Here's how the part is built. I have some questions about the finished solid (model axes, mm). Face numbers are marked on the shaded views. A direction names the side the tool comes from. Coordinates: 2 decimals unless noted, no trailing zeros. Write each loop counter-clockwise with the first axis right and the second up, starting at its lowest first coordinate (ties: lowest second). Pieces come first, ordered by that corner, then holes.
(1) Which directions (+Z, -Z, +X, -X, +Y, -Y) give clear straight access to the entire face, cutting with the end or side of a thin tool? Please do the marked faces 1, 2 and 3.
(2) Imagine slicing it at C-C, the plane y = -7.5. List the corners of the cut face in (x, z) for me (3 decimals).
(3) Imagine slicing it at D-D, the plane x = 2. List the corners of the cut face in (y, z) for me.
(4) Imagine slicing it at A-A, the plane y = 16.5. List the corners of the cut face in (x, z) for me.
(5) Thinking about a two-plate mould opening in Z: for the marked faces 4, 5, 6 and 7, which applies, released by +Z, released by -Z, zero draft, split by the parting line, or undercut?
(6) Please list where these lines run through material, in increasing order: probe 1 along Y at (x, z) = (0.25, 3.5); probe 2 along Y at (x, z) = (0, 3.65); probe 3 along Z at (x, y) = (0.6, 16.5).
(7) Imagine slicing it at B-B, the plane z = 4.75. List the corners of the cut face in (x, y) for me.
(8) For pin 1 Ø3 at (y, z) = (15.5, 4.5) entering from -X; pin 2 Ø0.8 at (x, z) = (-2, 2) entering from +Y, each with a flat end and sliding along its axis, tell me the tip position at first contact or that it passes through.
```python
from build123d import *

# Parameters (mm, degrees)
BOSS_EXTRUDE1_DEPTH = 6
SKETCH2_R           = 1.6
CUT_EXTRUDE1_DEPTH  = 22.644860822
CUT_EXTRUDE2_DEPTH  = 2.5
SKETCH4_R           = 1.1
CUT_EXTRUDE3_DEPTH  = 22.828879953
CUT_EXTRUDE4_DEPTH  = 22.828879953
FILLET1_R           = 2


with BuildPart() as part:
    # Sketch1 → Boss-Extrude1 (new body)
    with BuildSketch(Plane.XY):
        Polygon((-1, 12.5), (-1, 20.5), (1, 20.5), (1, 12.5), (3.5, 12.5), (3.5, -12.5), (-3.5, -12.5), (-3.5, 12.5), align=None)
    extrude(amount=BOSS_EXTRUDE1_DEPTH)

    # Sketch2 → Cut-Extrude1 (cut, through all)
    with BuildSketch(Plane.XY.offset(6)):
        with Locations((0, -7.5)):
            Circle(SKETCH2_R)
    extrude(amount=-CUT_EXTRUDE1_DEPTH, mode=Mode.SUBTRACT)

    # Sketch3 → Cut-Extrude2 (cut)
    with BuildSketch(Plane(origin=(0, 0, 0), x_dir=(-1, 0, 0), z_dir=(0, 0, -1))):
        Polygon((0, -4.295706006), (-2.775, -5.897853003), (-2.775, -9.102146997), (0, -10.704293994), (2.775, -9.102146997), (2.775, -5.897853003), align=None)
    extrude(amount=-CUT_EXTRUDE2_DEPTH, mode=Mode.SUBTRACT)

    # Sketch4 → Cut-Extrude3 (cut, through all)
    with BuildSketch(Plane.ZY.offset(1)):
        with Locations(Location((3, 16.5, 0), (0, 0, 270))):
            Circle(SKETCH4_R)
    extrude(amount=-CUT_EXTRUDE3_DEPTH, mode=Mode.SUBTRACT)

    # Sketch5 → Cut-Extrude4 (cut, through all)
    with BuildSketch(Plane.ZY.offset(1)):
        with BuildLine():
            Line((6, 20.5), (3, 20.5))
            ThreePointArc((3, 20.5), (4.645751311, 20.145751311), (6, 19.145751311))
            Line((6, 19.145751311), (6, 20.5))
        make_face()
        with BuildLine():
            Line((0, 20.5), (0, 19.145751311))
            ThreePointArc((0, 19.145751311), (1.354248689, 20.145751311), (3, 20.5))
            Line((3, 20.5), (0, 20.5))
        make_face()
    extrude(amount=-CUT_EXTRUDE4_DEPTH, mode=Mode.SUBTRACT)

    # Fillet1
    fillet1_edges = [part.edges().sort_by_distance(p)[0] for p in [
        (3.5, -12.5, 3),
        (-3.5, -12.5, 3),
    ]]
    fillet(fillet1_edges, radius=FILLET1_R)


solid = part.part
```
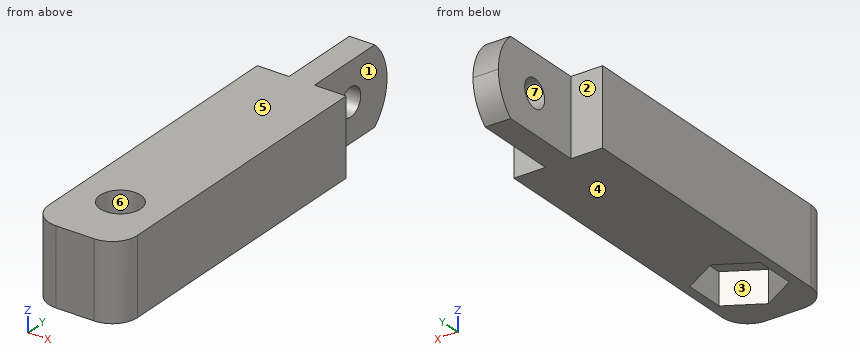
Recorded:
1. face 1: +Z, -Z, +X, +Y
1. face 2: +Z, -Z, -X, +Y
1. face 3: -Z
2. outline: (-3.5, 0) - (-2.775, 0) - (-2.775, 2.5) - (-1.6, 2.5) - (-1.6, 6) - (-3.5, 6) - close; (1.6, 2.5) - (2.775, 2.5) - (2.775, 0) - (3.5, 0) - (3.5, 6) - (1.6, 6) - close
3. outline: (-12.44, 0) - (-9.55, 0) - (-9.55, 2.5) - (-5.45, 2.5) - (-5.45, 0) - (12.5, 0) - (12.5, 6) - (-12.44, 6) - close
4. outline: (-1, 0) - (1, 0) - (1, 1.9) - (-1, 1.9) - close; (-1, 4.1) - (1, 4.1) - (1, 6) - (-1, 6) - close
5. face 4: released by -Z
5. face 5: released by +Z
5. face 6: zero draft
5. face 7: undercut
6. probe 1: y = -12.5 to -9.08, -5.92 to 15.52, 17.48 to 20.47
6. probe 2: y = -12.5 to -9.1, -5.9 to 15.61, 17.39 to 20.45
6. probe 3: z = 0 to 1.9, 4.1 to 6
7. outline: (-3.5, -10.5) arc R2 ccw to (-1.5, -12.5) - (1.5, -12.5) arc R2 ccw to (3.5, -10.5) - (3.5, 12.5) - (1, 12.5) - (1, 20.1) - (-1, 20.1) - (-1, 12.5) - (-3.5, 12.5) - close; hole circle Ø3.2 at (0, -7.5)
8. pin 1: stops at x = -1
8. pin 2: stops at y = 12.5
